Geometry: see drawing. Coordinates: mm, zero at the bounding-box minimum. A direction names the side the tool comes from. Coordinates: 2 decimals unless noted, no trailing zeros. Write each loop counter-clockwise with the first axis right and the second up, starting at its lowest first coordinate (ties: lowest second). Pieces come first, ordered by that corner, then holes. Notation, with made-up numbers: (72.5, -9) -> (91.5, -9) arc R16 cw to (91.5, 12) -> close; hole circle Ø7 at (-27, 79.25). An arc over 180 degrees is marked (long way). Use one line per item in the form item = value. Start each with the question number.
(1) Cut plane D-D on z = 10.5. Return the cut outline in (x, y).
(2) Ray query, line 1 along Z through (x, y) = (2.05, 10.5); line 2 along Z through (x, y) = (1.6, 18.5); line 3 along Y through (x, z) = (0.8, 22.25). Return the intervals inside material, ascending.
(3) Cut plane C-C on x = 0.5. Return the cut outline in (y, z).
(4) Set-up query: the marked faces 1, 2 and 3. Return all of +Z, -Z, +X, -X, +Y, -Y with unobstructed straight access to the full face (end or side cutting, diameter ignored); none if empty.
(5) First-contact query: pin 1 (1 mm diameter, centred on x = 2.5, y = 2.5, fed in from +Z); pin 2 (1 mm diameter, centred on x = 1, z = 19.5, fed in from +Y); pin 3 (0.7 mm diameter, centred on x = 2.5, y = 8, fed in from +Z). Flat tips, straight axial feed; report the tip coordinate or a pass-through.
(6) Pull-direction query (Z, two-part tool) for the marked faces 4, 5 and 6; classes: released by +Z, released by -Z, zero draft, split by the parting line, or undercut.
(7) Cut plane B-B on z = 3.25. Return the cut outline in (x, y).
(8) Cut plane A-A on y = 20. Return the cut outline in (x, z).
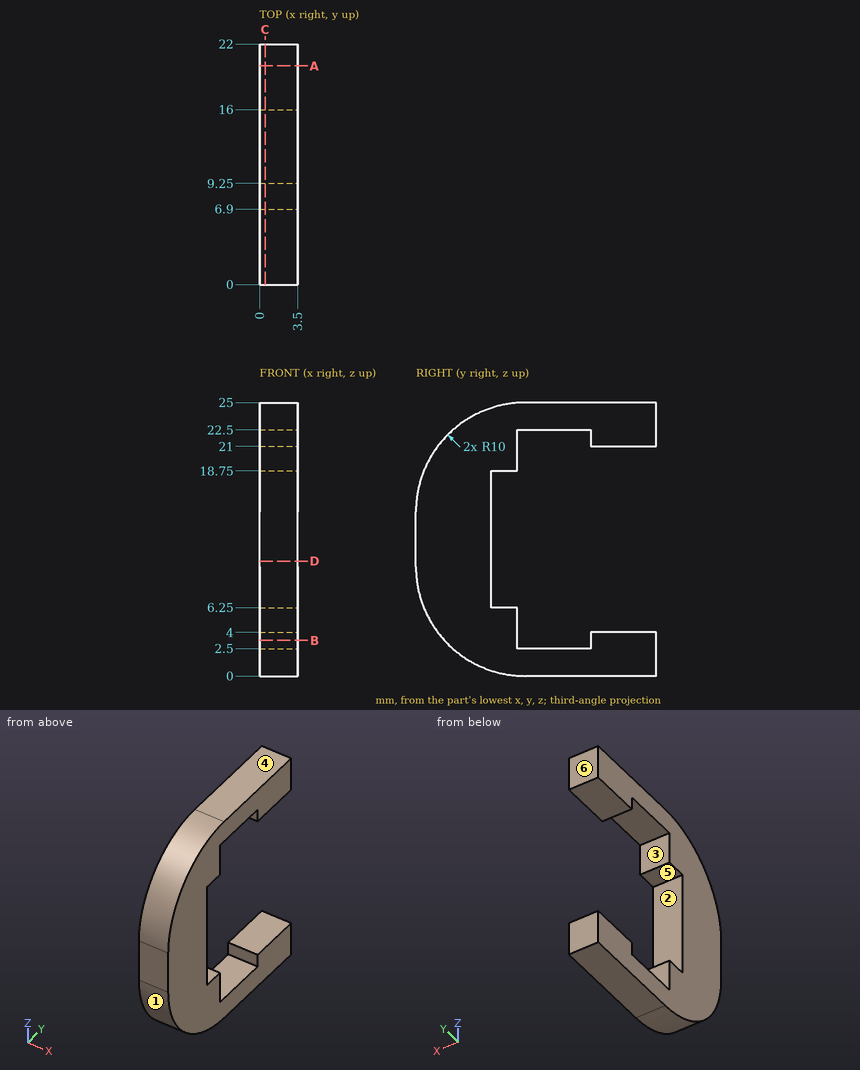
Values:
q1.outline = (0, 0) -> (3.5, 0) -> (3.5, 6.9) -> (0, 6.9) -> close
q2.line_1 = 0 to 2.5, 22.5 to 25
q2.line_2 = 0 to 4, 21 to 25
q2.line_3 = 3.11 to 9.25, 16 to 22
q3.outline = (0, 10) arc R10 ccw to (10, 0) -> (22, 0) -> (22, 4) -> (16, 4) -> (16, 2.5) -> (9.25, 2.5) -> (9.25, 6.25) -> (6.9, 6.25) -> (6.9, 18.75) -> (9.25, 18.75) -> (9.25, 22.5) -> (16, 22.5) -> (16, 21) -> (22, 21) -> (22, 25) -> (10, 25) arc R10 ccw to (0, 15) -> close
q4.face_1 = -Z, +X, -X, -Y
q4.face_2 = +X, -X, +Y
q4.face_3 = +X, -X
q5.pin_1 = 22.14
q5.pin_2 = 9.25
q5.pin_3 = 24.86
q6.face_4 = released by +Z
q6.face_5 = undercut
q6.face_6 = zero draft
q7.outline = (0, 2.62) -> (3.5, 2.62) -> (3.5, 9.25) -> (0, 9.25) -> close; (0, 16) -> (3.5, 16) -> (3.5, 22) -> (0, 22) -> close
q8.outline = (0, 0) -> (3.5, 0) -> (3.5, 4) -> (0, 4) -> close; (0, 21) -> (3.5, 21) -> (3.5, 25) -> (0, 25) -> close
